CAD build for the part. Positions are in the model's coordinates, mm. A direction names the side the tool comes from. Coordinates: 2 decimals unless noted, no trailing zeros. Order: outer loops, then holes, each group sorted by start corner. A loop starts at its lowest first (then second) coordinate and runs counter-clockwise, first axis right, second up. Notation, with made-up numbers: M -27.5,14 L 9.5,14 A20 cw 9.5,38 Z; hole C -28.5,-22.5 d1. An arc over 180 degrees is marked long. One line per item, written item: value.
from build123d import *

# Parameters (mm, degrees)
SKETCH_1_W          = 53
SKETCH_1_H          = 145
EXTRUDE_1_DEPTH     = 1.5
EXTRUDE_2_DEPTH     = 65
SKETCH_3_W          = 50
SKETCH_3_H          = 1.5
EXTRUDE_3_DEPTH     = 10
SKETCH_4_W          = 3
SKETCH_4_H          = 22
CUT_EXTRUDE_1_DEPTH = 100
SKETCH_5_W          = 55
SKETCH_5_H          = 10
CUT_EXTRUDE_2_DEPTH = 100


with BuildPart() as part:
    # Эскиз1 → Бобышка-Вытянуть1 (new body)
    with BuildSketch(Plane.XY):
        with Locations((26.5, 72.5)):
            Rectangle(SKETCH_1_W, SKETCH_1_H)
    extrude(amount=EXTRUDE_1_DEPTH)

    # Эскиз2 → Бобышка-Вытянуть2 (add)
    with BuildSketch(Plane.XY.offset(1.5)):
        Polygon((1.5, 145), (1.5, 1.5), (51.5, 1.5), (51.5, 145), (53, 145), (53, 0), (0, 0), (0, 145), align=None)
    extrude(amount=EXTRUDE_2_DEPTH)

    # Эскиз3 → Бобышка-Вытянуть3 (add)
    with BuildSketch(Plane.XY.offset(1.5)):
        with Locations((26.5, 144.25)):
            Rectangle(SKETCH_3_W, SKETCH_3_H)
    extrude(amount=EXTRUDE_3_DEPTH)

    # Эскиз4 → Вырез-Вытянуть1 (cut)
    with BuildSketch(Plane(origin=(53, 0, 0), x_dir=(0, 0, -1), z_dir=(1, 0, 0))):
        with Locations((-3, 114)):
            Rectangle(SKETCH_4_W, SKETCH_4_H)
        with Locations((-3, 31)):
            Rectangle(SKETCH_4_W, SKETCH_4_H)
    extrude(amount=-CUT_EXTRUDE_1_DEPTH, mode=Mode.SUBTRACT)

    # Эскиз5 → Вырез-Вытянуть2 (cut)
    with BuildSketch(Plane(origin=(53, 0, 0), x_dir=(0, 0, -1), z_dir=(1, 0, 0))):
        with Locations((-39, 140)):
            Rectangle(SKETCH_5_W, SKETCH_5_H)
    extrude(amount=-CUT_EXTRUDE_2_DEPTH, mode=Mode.SUBTRACT)


solid = part.part
Q1. Slice it at B-B (z = 10). List the corners of the cut face in (x, y), plus the area to 3 significant figures.
Recorded:
outline: M 0,0 L 53,0 L 53,145 L 0,145 Z; hole M 1.5,1.5 L 51.5,1.5 L 51.5,143.5 L 1.5,143.5 Z
area: 585 mm^2
Q2. Slice it at C-C (x = 8). List the corners of the cut face in (y, z).
Recorded:
outline: M 0,0 L 145,0 L 145,11.5 L 143.5,11.5 L 143.5,1.5 L 1.5,1.5 L 1.5,66.5 L 0,66.5 Z
Q3. Drill centre lines: line 1 along X through (y, z) = (89, 35); line 2 along Z through (x, y) = (45, 9.5). Where is each one in solid material? Low to high.
Recorded:
line 1: x = 0 to 1.5, 51.5 to 53
line 2: z = 0 to 1.5
Q4. Which spindle directions (+Z, -Z, +X, -X, +Y, -Y) get a long thin tool onto all of the face, cutting with end or side? Do faces 4 (the face through (1.5, 73, 34)), 5 (the face through (26, 144, 11.5)), 6 (the face through (26, 145, 6)). Say none if no direction does.
Recorded:
face 4: +Z
face 5: +Z, +X, -X, +Y
face 6: +Z, -Z, +X, -X, +Y
Q5. Pin check, flat tips, straight feed: pin 1 Ø1 at (x, z) = (34, 17) entering from +Y; pin 2 Ø10 at (x, y) = (37, 89) entering from +Z; pin 3 Ø1.2 at (x, z) = (52.5, 37.5) entering from +Y. Stop position of each tip, or through.
Recorded:
pin 1: stops at y = 1.5
pin 2: stops at z = 1.5
pin 3: stops at y = 135
Q6. Slice it at A-A (y = 107.5). List the corners of the cut face in (x, z), plus the area to 4 significant figures.
Recorded:
outline: M 0,0 L 53,0 L 53,1.5 L 0,1.5 Z; M 0,4.5 L 1.5,4.5 L 1.5,66.5 L 0,66.5 Z; M 51.5,4.5 L 53,4.5 L 53,66.5 L 51.5,66.5 Z
area: 265.5 mm^2
Q7. Slice it at D-D (z = 37.5). List the corners of the cut face in (x, y), plus the area to 3 significant figures.
Recorded:
outline: M 0,0 L 53,0 L 53,135 L 51.5,135 L 51.5,1.5 L 1.5,1.5 L 1.5,135 L 0,135 Z
area: 480 mm^2
Q8. Mould opens along X. For faces 1 (the face through (53, 74, 33)), 2 (the face through (27, 0, 33)), 3 (the face through (26, 73, 1.5)) say: released by +X, released by -X, zero draft, split by the parting line, or undercut.
Recorded:
face 1: released by +X
face 2: zero draft
face 3: undercut
